Autodesk Inventor part; units mm, degrees
ref_plane "YZ Plane" through (0, 0, 0) normal (1, 0, 0) x (0, 1, 0)
ref_plane "XZ Plane" through (0, 0, 0) normal (0, 1, 0) x (-1, 0, 0)
ref_plane "XY Plane" through (0, 0, 0) normal (0, 0, 1) x (1, 0, 0)
sketch "Sketch1" plane through (0, 0, 0) normal (0, 0, 1) x (1, 0, 0)
  arc A0 (670.9948, -199.4141) -> (0, 0) centre (254.9219, -370.8299) ccw
  arc A1 (657.7848, -239.4141) -> (30, 0) centre (229.3296, -420.1103) ccw
  arc A2 (657.7848, -239.4141) -> (670.9948, -199.4141) centre (0, 0) ccw
  line L0 (0, 0) -> (30, 0)
  line L1 (657.7848, -239.4141) -> (0, 0)
  line L2 (-143.7228, 0) -> (862.3369, 0)
  point P0 (0, 0)
  dimension "d1" = 30
  dimension "d2" = 40
  dimension "d4" = 20
  dimension "d5" = 465
  dimension "d6" = 450
  dimension "d22" = 700
extrude "Extrusion1" add sketch "Sketch1" along normal blind 4 contours A2 A1 L2 A0 | L2 A1 L0 A0
sketch "Sketch2" plane through (0, 0, 4) normal (0, 0, 1) x (1, 0, 0)
  arc A0 (670.9948, -199.4141) -> (0, 0) centre (254.9219, -370.8299) ccw
  arc A1 (87.1309, 22.5434) -> (74.166, 50.9844) centre (0, 0) ccw
  line L0 (74.166, 50.9844) -> (0, 0)
  line L1 (0, 0) -> (87.1309, 22.5434)
  line L2 (0, 0) -> (30, 0)
  point P0 (78.8927, 43.3122)
  point P1 (0, 0)
  point P2 (0, 0)
  dimension "d9" = 90
  dimension "d16" = 20
extrude "Extrusion2" add sketch "Sketch2" against normal blind 4
sketch "Sketch4" plane through (0, 0, 4) normal (0, 0, 1) x (1, 0, 0)
  line L0 (86.0304, 22.2587) -> (87.1309, 22.5434)
  line L1 (74.166, 50.9844) -> (0, 0)
  line L2 (87.1309, 22.5434) -> (0, 0)
  line L3 (0, 0) -> (30, 0)
  arc A0 (86.0304, 22.2587) -> (30, 0) centre (229.3296, -420.1103) ccw
  line L4 (30, 0) -> (86.0304, 22.2587)
  point P0 (86.0304, 22.2587)
extrude "Extrusion4" cut sketch "Sketch4" against normal blind 10 contours A0 L3 L2
sketch "Sketch6" plane through (0, 0, 4) normal (0, 0, 1) x (1, 0, 0)
  circle A0 centre (71.4659, 35.9531) radius 1.5
  circle A1 centre (76.6234, 22.9969) radius 1.5
  circle A2 centre (37.1637, 14.7938) radius 1.5
  line L0 (0, 0) -> (87.1309, 22.5434)
  line L1 (37.1637, 14.7938) -> (0, 0)
  line L2 (0, 0) -> (71.4659, 35.9531)
  line L3 (74.166, 50.9844) -> (0, 0)
  line L4 (76.6234, 22.9969) -> (0, 0)
  circle A3 centre (264.574, 53.8573) radius 1.5
  circle A4 centre (260.1726, 72.1818) radius 1.5
  line L5 (261.3927, 67.6302) -> (0, 0)
  line L6 (264.574, 53.8573) -> (0, 0)
  circle A5 centre (281.2279, 70.1567) radius 1.5
  circle A6 centre (285.6292, 51.8321) radius 1.5
  line L7 (264.574, 53.8573) -> (260.1726, 72.1818)
  line L8 (281.2279, 70.1567) -> (260.1726, 72.1818)
  line L9 (281.2279, 70.1567) -> (285.6292, 51.8321)
  line L10 (285.6292, 51.8321) -> (264.574, 53.8573)
  line L11 (260.1726, 72.1818) -> (0, 0)
  dimension "d23" = 7.2
  dimension "d24" = 2.2
  dimension "d25" = 7.8
  dimension "d26" = 80
  dimension "d27" = 80
  dimension "d28" = 40
  dimension "d29" = 3
  dimension "d30" = 3
  dimension "d31" = 3
  dimension "d34" = 3
  dimension "d35" = 3
  dimension "d36" = 3
  dimension "d38" = 270
  dimension "d39" = 270
  dimension "d40" = 109
  dimension "d41" = 3
  dimension "d42" = 3
  dimension "d43" = 20
  dimension "d47" = 1
  dimension "d48" = 270
extrude "Extrusion6" cut sketch "Sketch6" against normal blind 10 from surface at 0 contours A0 | A1 | A2 | L6 L10 A3 | A3 L7 L6 | L11 L7 A4 | A4 L8 L11 | A3 L10 L7 | L7 L8 A4 | L10 L9 A6 | A6 L9 L10 | L8 L9 A5 | A5 L9 L8
sketch "Sketch7" plane through (0, 0, 4) normal (0, 0, 1) x (1, 0, 0)
  line L0 (87.1309, 22.5434) -> (0, 0)
  circle A0 centre (0, 0) radius 15
  dimension "d44" = 30
extrude "Extrusion7" cut sketch "Sketch7" against normal blind 10
sketch "Sketch8" plane through (0, 0, 4) normal (0, 0, 1) x (1, 0, 0)
  arc A0 (78.8927, 43.3122) -> (74.166, 50.9844) centre (0, 0) ccw
  line L0 (74.166, 50.9844) -> (0, 0)
  line L1 (12.361, 8.4974) -> (74.166, 50.9844)
  line L2 (0, 0) -> (82.5313, 50.9844)
  line L3 (82.5313, 50.9844) -> (74.166, 50.9844)
  point P0 (76.568, 47.3005)
  dimension "d49" = 2.8
extrude "Extrusion8" cut sketch "Sketch8" against normal blind 10 contours L2 L0 A0
sketch "Sketch9" plane through (0, 0, 4) normal (0, 0, 1) x (1, 0, 0)
  line L0 (14.5218, 3.7572) -> (87.1309, 22.5434)
  line L1 (87.1309, 22.5434) -> (14.5218, 3.7572)
  arc A0 (14.688, 3.0434) -> (14.5218, 3.7572) centre (0, 0) ccw
  line L2 (14.688, 3.0434) -> (88.1281, 18.2602)
  arc A1 (88.1281, 18.2602) -> (87.1309, 22.5434) centre (0, 0) ccw
  line L3 (14.688, 3.0434) -> (0, 0)
  line L4 (0, 0) -> (14.5218, 3.7572)
  arc A2 (78.8927, 43.3122) -> (76.568, 47.3005) centre (0, 0) ccw
  dimension "d52" = 2.8
extrude "Extrusion9" add sketch "Sketch9" against normal blind 4 contours L0 A1 L2 A0
properties part number "spoke3"
The listing builds one solid part. Answer for the finished solid, in the listing's coordinates (mm). A direction names the side the tool comes from. Give positions to 0.01 mm unless a question says otherwise; leave off trailing zeros. Order: outer loops, then holes, each group sorted by start corner. A loop starts at its lowest first (then second) coordinate and runs counter-clockwise, first axis right, second up. Notation, with made-up numbers: (15, 35.5) - (35, 35.5) arc R23 cw to (35, 56.5) - close; hole circle Ø6 at (55, -20.75). An arc over 180 degrees is marked (long way). Use one line per item in the form item = value.
1) For faces 1 (the cylindrical face through (664.783, -219.233, 1.972)), 2 (the flat face through (50.894, 10.545, 2.028)), determine the directions among +Z, -Z, +X, -X, +Y, -Y from which every point of the face is accessible in a straight line to the end or side of a thin tool.
Verdict:
face_1 = +Z, -Z, +X, -Y
face_2 = +Z, -Z, -Y
2) Consider probe 1 along Y at (x, z) = (268, 1.1); probe 2 along X at (y, z) = (-212.5, 0.4); probe 3 along X at (y, z) = (-107.5, 3.2). Determine where each line is inside the solid, lowest interval first. Write a range as [from, to].
Verdict:
probe_1 = [43.28, 78.98]
probe_2 = [645.41, 666.97]
probe_3 = [573.57, 619.83]
3) The mould has two halves that part along X. Classify faces 3 (the flat face through (413, 15, 4)), 4 (the cylindrical face through (418.963, 4.465, 1.972)), 5 (the flat face through (44.218, 27.316, 2.028)): released by +X, released by -X, zero draft, split by the parting line, or undercut.
Verdict:
face_3 = zero draft
face_4 = undercut
face_5 = released by -X
4) Each of these flat-tipped pins is pushed along its axis until it touches: pin 1 (1.8 mm diameter, centred on x = 37.16, y = 14.79, fed in from -Z) (3 decimals); pin 2 (5 mm diameter, centred on x = 281.23, y = 70.16, fed in from +Z); pin 3 (1.5 mm diameter, centred on y = -126.5, z = 0.5, fed in from +X); pin 4 (1 mm diameter, centred on x = 521.5, z = 3, fed in from +Y). Where does it stop, or does it pass through?
Verdict:
pin_1 = through
pin_2 = 4
pin_3 = 633.3
pin_4 = -7.92
5) Find section C-C on y = -182. Determine the outline of the cut face in (x, z).
Verdict:
outline = (628.74, 0) - (663.39, 0) - (663.39, 4) - (628.74, 4) - close
6) Find section A-A on z = 0.8. Determine the outline of the cut face in (x, y), and give its area (3 significant figures).
Verdict:
outline = (12.76, 7.88) arc R15 cw to (14.52, 3.76) arc R14.98 cw to (14.69, 3.04) - (88.13, 18.26) arc R90.02 ccw to (87.13, 22.54) arc R90 ccw to (87.11, 22.61) arc R465 cw to (657.78, -239.41) arc R700.04 ccw to (670.99, -199.41) arc R450 ccw to (78.89, 43.31) arc R90 ccw to (76.57, 47.3) - close; hole circle Ø3 at (37.16, 14.79); hole circle Ø3 at (71.47, 35.95); hole circle Ø3 at (76.62, 23); hole circle Ø3 at (260.17, 72.18); hole circle Ø3 at (264.57, 53.86); hole circle Ø3 at (281.23, 70.16); hole circle Ø3 at (285.63, 51.83)
area = 25,900 mm^2
7) Find section B-B on x = 101.5. Determine the outline of the cut face in (y, z), and give its area (3 significant figures).
Verdict:
outline = (26.97, 0) - (52.21, 0) - (52.21, 4) - (26.97, 4) - close
area = 101 mm^2
